Verification items for the finished model (mm, model axes). Face numbers are marked on the shaded views. A direction names the side the tool comes from. Round coordinates to 2 decimals unless told otherwise and drop trailing zeros. Loops run counter-clockwise (first coordinate to the right, second up) from the corner with the lowest first, then second, coordinate; pieces in that order, holes last.
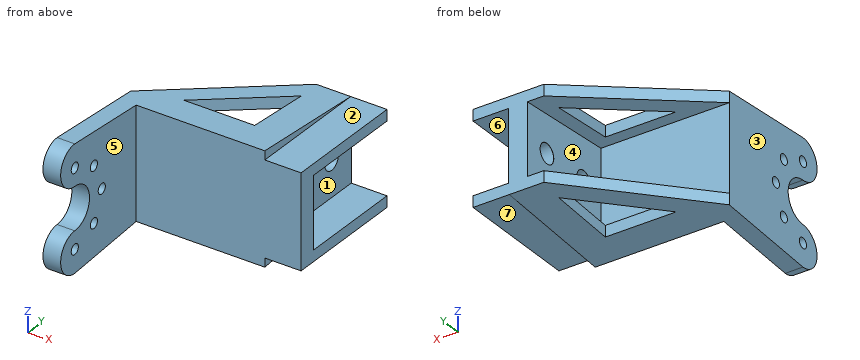
from build123d import *

# Parameters (mm, degrees)
EXTRUDE_1_DEPTH                  = 35
SKETCH_6_R                       = 6
CUT_EXTRUDE_2_DEPTH              = 103.2
SKETCH_7_R                       = 5.75
EXTRUDE_3_DEPTH                  = 103.2
CUT_EXTRUDE_3_REACH              = 88.478
M2_5_CLEARANCE_HOLE1_D           = 2.9
M2_5_CLEARANCE_HOLE1_CSINK_D     = 2.95
M2_5_CLEARANCE_HOLE1_CSINK_ANGLE = 90
SKETCH_16_W                      = 20.2
SKETCH_16_H                      = 20.2
CUT_EXTRUDE_5_DEPTH              = 30
SKETCH_15_W                      = 20.5
SKETCH_15_H                      = 35
CUT_EXTRUDE_6_DEPTH              = 4.25
SKETCH_17_W                      = 20.5
SKETCH_17_H                      = 35
CUT_EXTRUDE_7_DEPTH              = 4.25
CUT_EXTRUDE_8_REACH              = 126.363
CUT_EXTRUDE_9_DEPTH              = 36.25
CUT_EXTRUDE_10_DEPTH             = 36.25
CUT_EXTRUDE_12_DEPTH             = 87.477815158
CUT_EXTRUDE1_START               = -51.6
SKETCH1_W                        = 50
SKETCH1_H                        = 80
CUT_EXTRUDE1_DEPTH               = 51.6
M5_CLEARANCE_HOLE2_D             = 5.5
M5_CLEARANCE_HOLE2_CSINK_D       = 5.55
M5_CLEARANCE_HOLE2_CSINK_ANGLE   = 90


with BuildPart() as part:
    # 草图1 → 凸台-拉伸1 (new body)
    with BuildSketch(Plane.XY):
        Polygon((51.6, -0.076277531), (51.6, 29.923722469), (20, 59.923722469), (-20, 59.923722469), (-51.6, 29.923722469), (-51.6, -0.076277531), align=None)
    extrude(amount=EXTRUDE_1_DEPTH)

    # 草图6 → 切除-拉伸2 (cut)
    with BuildSketch(Plane.ZY.offset(51.6)):
        with Locations((17.5, -0.076277531)):
            Circle(SKETCH_6_R)
    extrude(amount=-CUT_EXTRUDE_2_DEPTH, mode=Mode.SUBTRACT)

    # 草图7 → 凸台-拉伸3 (add)
    with BuildSketch(Plane.ZY.offset(51.6)):
        with Locations((5.75, -0.076277531)):
            Circle(SKETCH_7_R)
        with Locations((29.25, -0.076277531)):
            Circle(SKETCH_7_R)
    extrude(amount=-EXTRUDE_3_DEPTH)

    # 切除-拉伸3: up to this face of the body (flat: up to its plane)
    cut_extrude_3_end = Plane(part.part.faces().sort_by_distance((0, 26.308161829, 0))[0])
    # 草图8 → 切除-拉伸3 (cut, up to the picked face)
    with BuildSketch(Plane.XY.offset(35), mode=Mode.PRIVATE) as cut_extrude_3_sk1:
        Polygon((-46.6, -0.076277531), (-46.6, 24.923722469), (46.6, 24.923722469), (46.6, -0.076277531), (46.6, -12.111349377), (-46.6, -12.111349377), align=None)
    cut_extrude_3_tool1 = split(extrude(cut_extrude_3_sk1.sketch, amount=-CUT_EXTRUDE_3_REACH, mode=Mode.PRIVATE), bisect_by=cut_extrude_3_end, keep=Keep.BOTH, mode=Mode.PRIVATE)
    add(cut_extrude_3_tool1.solids().sort_by(Axis((0, 6.406187, 35), (0, 0, -1)))[0], mode=Mode.SUBTRACT)

    # M2.5 Clearance Hole1 (through all)
    with Locations(Plane(origin=(51.6, 0, 0), x_dir=(0, 0, -1), z_dir=(1, 0, 0))):
        with Locations((-28.5, -0.076277531), (-25.278174593, 7.701897062), (-17.5, 10.923722469), (-9.721825407, 7.701897062), (-6.5, -0.076277531)):
            CounterSinkHole(M2_5_CLEARANCE_HOLE1_D / 2, M2_5_CLEARANCE_HOLE1_CSINK_D / 2, counter_sink_angle=M2_5_CLEARANCE_HOLE1_CSINK_ANGLE)

    # 草图16 → 切除-拉伸5 (cut)
    with BuildSketch(Plane(origin=(0, 59.923722469, 0), x_dir=(1, 0, 0), z_dir=(0, 1, 0))):
        with Locations((0, -17.5)):
            Rectangle(SKETCH_16_W, SKETCH_16_H)
    extrude(amount=-CUT_EXTRUDE_5_DEPTH, mode=Mode.SUBTRACT)

    # 草图15 → 切除-拉伸6 (cut)
    with BuildSketch(Plane.XY.offset(35)):
        with Locations((0, 42.423722469)):
            Rectangle(SKETCH_15_W, SKETCH_15_H)
    extrude(amount=-CUT_EXTRUDE_6_DEPTH, mode=Mode.SUBTRACT)

    # 草图17 → 切除-拉伸7 (cut)
    with BuildSketch(Plane(origin=(0, 0, 0), x_dir=(-1, 0, 0), z_dir=(0, 0, -1))):
        with Locations((0, 42.423722469)):
            Rectangle(SKETCH_17_W, SKETCH_17_H)
    extrude(amount=-CUT_EXTRUDE_7_DEPTH, mode=Mode.SUBTRACT)

    # 切除-拉伸8: up to this face of the body (flat: up to its plane)
    cut_extrude_8_end = Plane(part.part.faces().sort_by_distance((-51.6, 14.183980779, 17.5))[0])
    # 草图20 → 切除-拉伸8 (cut, up to the picked face)
    with BuildSketch(Plane(origin=(51.6, 0, 0), x_dir=(0, 0, -1), z_dir=(1, 0, 0)), mode=Mode.PRIVATE) as cut_extrude_8_sk1:
        Polygon((-30.75, 59.923722469), (-35, 59.923722469), (-35, -0.076277531), align=None)
    cut_extrude_8_tool1 = split(extrude(cut_extrude_8_sk1.sketch, amount=-CUT_EXTRUDE_8_REACH, mode=Mode.PRIVATE), bisect_by=cut_extrude_8_end, keep=Keep.BOTH, mode=Mode.PRIVATE)
    # 草图20 → 切除-拉伸8 (cut, up to the picked face)
    with BuildSketch(Plane(origin=(51.6, 0, 0), x_dir=(0, 0, -1), z_dir=(1, 0, 0)), mode=Mode.PRIVATE) as cut_extrude_8_sk2:
        Polygon((0, -0.076277531), (0, 59.923722469), (-4.25, 59.923722469), align=None)
    cut_extrude_8_tool2 = split(extrude(cut_extrude_8_sk2.sketch, amount=-CUT_EXTRUDE_8_REACH, mode=Mode.PRIVATE), bisect_by=cut_extrude_8_end, keep=Keep.BOTH, mode=Mode.PRIVATE)
    add(cut_extrude_8_tool1.solids().sort_by(Axis((51.6, 39.923722, 33.583333), (-1, 0, 0)))[0], mode=Mode.SUBTRACT)
    add(cut_extrude_8_tool2.solids().sort_by(Axis((51.6, 39.923722, 1.416667), (-1, 0, 0)))[0], mode=Mode.SUBTRACT)

    # 草图21 → 切除-拉伸9 (cut)
    with BuildSketch(Plane(origin=(51.6, 0, 0), x_dir=(0, 0, -1), z_dir=(1, 0, 0))):
        Polygon((-27.6, 59.923722469), (-29.725, 29.923722469), (-5.275, 29.923722469), (-7.4, 59.923722469), align=None)
    extrude(amount=-CUT_EXTRUDE_9_DEPTH, mode=Mode.SUBTRACT)

    # 草图22 → 切除-拉伸10 (cut)
    with BuildSketch(Plane.ZY.offset(51.6)):
        Polygon((29.725, 29.923722469), (27.6, 59.923722469), (7.4, 59.923722469), (5.275, 29.923722469), align=None)
    extrude(amount=-CUT_EXTRUDE_10_DEPTH, mode=Mode.SUBTRACT)

    # 草图25 → 切除-拉伸12 (cut, through all)
    with BuildSketch(Plane.XY):
        Polygon((39.35, 33.923722469), (19.35, 33.923722469), (19.35, 52.911064241), align=None)
        Polygon((-19.35, 52.911064241), (-39.35, 33.923722469), (-19.35, 33.923722469), align=None)
    extrude(amount=CUT_EXTRUDE_12_DEPTH, mode=Mode.SUBTRACT)

    # Sketch1 → Cut-Extrude1 (cut)
    with BuildSketch(Plane(origin=(51.6, 0, 0), x_dir=(0, 0, -1), z_dir=(1, 0, 0)).offset(CUT_EXTRUDE1_START)):
        with Locations((-17.5, 29.923722469)):
            Rectangle(SKETCH1_W, SKETCH1_H)
    extrude(amount=CUT_EXTRUDE1_DEPTH, mode=Mode.SUBTRACT)

    # M5 Clearance Hole2 (through all)
    with Locations(Plane.ZY.offset(15.35)):
        with Locations((17.5, 36.923722469), (17.5, 51.923722469)):
            CounterSinkHole(M5_CLEARANCE_HOLE2_D / 2, M5_CLEARANCE_HOLE2_CSINK_D / 2, counter_sink_angle=M5_CLEARANCE_HOLE2_CSINK_ANGLE)


solid = part.part
1. Section check C-C (x = -7). Enter the section's corners in (y, z), then the cut area to 4 significant figures.
2. Section check D-D (x = -30.5). Enter the section's corners in (y, z) (3 decimals), then the cut area to 3 significant figures.
3. Scan lines: L1, parallel to Y at x = -13.95, z = 17.5; L2, parallel to Y at x = -49.6, z = 17.5; L3, parallel to X at y = 7, z = 17. Record each from-to range of solid material in increasing order.
4. Section check B-B (y = 43). Enter the section's corners in (x, z), then the cut area to 3 significant figures.
5. Section check A-A (z = 17.5). Enter the section's corners in (x, y) (3 decimals).
6. Release check for a two-part mould opening along Z. For the marked faces 1, 2 and 3 record: released by +Z, released by -Z, zero draft, split by the parting line, or undercut.
7. Tool access check on the marked faces 4, 5, 6 and 7. Record the directions out of +Z, -Z, +X, -X, +Y, -Y that give a thin tool (end or side, any length) a straight path to the whole face; none if there is none.
8. Gauge pin test, flat ends, axial feed: P1, Ø3, axis at x = -34.5, z = 11, coming from the -Y side; P2, Ø16, axis at y = 48.5, z = 16.5, coming from the +X side; P3, Ø4, axis at x = -23.5, y = 24.5, coming from the -Z side; P4, Ø2.5, axis at y = -0.08, z = 6.5, coming from the +X side. Record the tip position at first contact, or that the pin passes through.
Taken from the geometry:
1. outline: (24.92, 4.25) - (59.92, 4.25) - (59.92, 7.4) - (29.92, 7.4) - (29.92, 27.6) - (59.92, 27.6) - (59.92, 30.75) - (24.92, 30.75) - close
1. area: 321.5 mm2
2. outline: (24.924, 1.771) - (33.924, 2.408) - (33.924, 5.558) - (29.924, 5.275) - (29.924, 29.725) - (33.924, 29.442) - (33.924, 32.592) - (24.924, 33.229) - close; (42.326, 3.003) - (49.955, 3.544) - (49.955, 6.694) - (42.326, 6.153) - close; (42.326, 28.847) - (49.955, 28.306) - (49.955, 31.456) - (42.326, 31.997) - close
2. area: 229 mm2
3. L1: y = 24.92 to 34.17, 39.67 to 49.17, 54.67 to 59.92
3. L2: y = 5.92 to 9.47, 12.37 to 29.92
3. L3: x = -51.6 to -46.6
4. outline: (-37.83, 3.05) - (-29.79, 3.05) - (-29.79, 6.2) - (-37.83, 6.2) - close; (-37.83, 28.8) - (-29.79, 28.8) - (-29.79, 31.95) - (-37.83, 31.95) - close; (-19.35, 3.05) - (-10.25, 3.05) - (-10.25, 4.25) - (0, 4.25) - (0, 7.4) - (-10.1, 7.4) - (-10.1, 27.6) - (0, 27.6) - (0, 30.75) - (-10.25, 30.75) - (-10.25, 31.95) - (-19.35, 31.95) - (-19.35, 28.8) - (-15.35, 28.8) - (-15.35, 6.2) - (-19.35, 6.2) - close
4. area: 291 mm2
5. outline: (-51.6, 5.924) - (-46.6, 5.924) - (-46.6, 9.474) - (-51.6, 9.474) - close; (-51.6, 12.374) - (-46.6, 12.374) - (-46.6, 24.924) - (0, 24.924) - (0, 29.924) - (-10.1, 29.924) - (-10.1, 34.174) - (-15.325, 34.174) - (-15.35, 34.149) - (-15.35, 29.924) - (-51.6, 29.924) - close; (-15.35, 39.699) - (-15.325, 39.674) - (-10.1, 39.674) - (-10.1, 49.174) - (-15.325, 49.174) - (-15.35, 49.149) - close; (-15.35, 54.699) - (-15.325, 54.674) - (-10.1, 54.674) - (-10.1, 59.924) - (-15.35, 59.924) - close
6. face 1: undercut
6. face 2: released by +Z
6. face 3: zero draft
7. face 4: -X
7. face 5: +Z, -Z, +X, -Y
7. face 6: +X, +Y
7. face 7: -Z, +X, +Y, -Y
8. P1: stops at y = 24.92
8. P2: stops at x = -10.1
8. P3: stops at z = 1.77
8. P4: passes through
